CAD build for the part. Positions are in the model's coordinates, mm. Face numbers are marked on the shaded views. Give positions to 0.01 mm unless a question says otherwise; leave off trailing zeros. Loops run counter-clockwise (first coordinate to the right, second up) from the corner with the lowest first, then second, coordinate; pieces in that order, holes last.
Item 1: Saw through at A-A on z = 1.15. Give the cut face in (x, y), plus the area to 3 significant figures.
Item 2: Saw through at B-B on y = -23.5. Give the cut face in (x, z), plus the area to 3 significant figures.
Item 3: Saw through at C-C on x = 16. Give the cut face in (y, z).
Item 4: Mould opens along X. For the marked faces 1 and 2 say: released by +X, released by -X, zero draft, split by the parting line, or undercut.
Item 5: Probe probe 1 along Y at (x, z) = (0, 2.9); probe 2 along Y at (x, z) = (5, 3.5); probe 3 along Y at (x, z) = (0, 4.3). List the from-to ranges inside material, lowest first.
Item 6: Saw through at D-D on y = -32.5. Give the cut face in (x, z), plus the area to 3 significant figures.
Item 7: Drop flat-ended pins along their axis: P1, Ø2, axis at y = -16.5, z = 0.5, coming from the -X side; P2, Ø2, axis at y = -14, z = 1, coming from the +X side; P3, Ø24, axis at x = -12.5, y = -14.5, coming from the +Z side. Give the stop position or say it passes through.
from build123d import *
from build123d import SkipClean  # not in build123d's __all__

# Parameters (mm, degrees)
F0_R      = 39.5
F1_DEPTH  = 2
F2_R      = 37.5
F2_R_2    = 35
F3_DEPTH  = 3
F4_R      = 4.1
F5_DEPTH  = 25
F6_R      = 6
F6_R_2    = 4.1
F7_DEPTH  = 2
F9_DEPTH  = 25
F11_DEPTH = 25


# Not quite as in the source:
# - after a boolean that leaves OpenCascade's solid faulty, fix() repairs it


with BuildPart() as f1:
    # F0 (on Top) → F1 (new body)
    with BuildSketch(Plane.XY):
        Circle(F0_R)
    extrude(amount=F1_DEPTH)

    # F2 (on face) → F3 (join)
    with BuildSketch(Plane.XY.offset(2)):
        Circle(F2_R)
        Circle(F2_R_2, mode=Mode.SUBTRACT)
    extrude(amount=F3_DEPTH)

    # F4 (on face) → F5 (cut)
    with BuildSketch(Plane.XY.offset(2)):
        Circle(F4_R)
    extrude(amount=-F5_DEPTH, mode=Mode.SUBTRACT)

    # F6 (on face) → F7 (join)
    with BuildSketch(Plane.XY.offset(2)):
        Circle(F6_R)
        Circle(F6_R_2, mode=Mode.SUBTRACT)
    extrude(amount=F7_DEPTH)

    # F8 (on face) → F9 (cut)
    with BuildSketch(Plane.XY.offset(2)):
        with BuildLine():
            Line((30.3108891325, 17.5), (0, 35))
            Line((0, 35), (0, 6))
            ThreePointArc((0, 6), (3, 5.1961524227), (5.1961524227, 3))
            Line((5.1961524227, 3), (30.3108891325, 17.5))
        make_face()
        with BuildLine():
            Line((0, -35), (30.3108891325, -17.5))
            Line((30.3108891325, -17.5), (5.1961524227, -3))
            ThreePointArc((5.1961524227, -3), (3, -5.1961524227), (0, -6))
            Line((0, -6), (0, -35))
        make_face()
        with BuildLine():
            ThreePointArc((30.3108891325, 17.5), (17.5, 30.3108891325), (0, 35))
            Line((0, 35), (30.3108891325, 17.5))
        make_face()
        with BuildLine():
            ThreePointArc((0, -35), (17.5, -30.3108891325), (30.3108891325, -17.5))
            Line((30.3108891325, -17.5), (0, -35))
        make_face()
        with BuildLine():
            Line((-5.1961524227, 3), (-30.3108891325, 17.5))
            Line((-30.3108891325, 17.5), (-30.3108891325, -17.5))
            Line((-30.3108891325, -17.5), (-5.1961524227, -3))
            ThreePointArc((-5.1961524227, -3), (-6, 0), (-5.1961524227, 3))
        make_face()
        with BuildLine():
            Line((-30.3108891325, -17.5), (-30.3108891325, 17.5))
            ThreePointArc((-30.3108891325, 17.5), (-35, 0), (-30.3108891325, -17.5))
        make_face()
    with SkipClean():  # cleaning this boolean's faces spoils the solid; the shape is the same uncleaned
        extrude(amount=-F9_DEPTH, mode=Mode.SUBTRACT)

    # F10 (on face) → F11 (cut)
    with BuildSketch(Plane.XY.offset(2)):
        with BuildLine():
            Line((-5, 9.7979589711), (-5, 29.5803989155))
            ThreePointArc((-5, 29.5803989155), (-15, 25.9807621135), (-23.1173769149, 19.1203264767))
            Line((-23.1173769149, 19.1203264767), (-5.9852813742, 9.2291065045))
            ThreePointArc((-5.9852813742, 9.2291065045), (-5.5, 9.5262794416), (-5, 9.7979589711))
        make_face()
        with BuildLine():
            ThreePointArc((10.9852813742, 0.5688524666), (11, 0), (10.9852813742, -0.5688524666))
            Line((10.9852813742, -0.5688524666), (28.1173769149, -10.4600724388))
            ThreePointArc((28.1173769149, -10.4600724388), (30, 0), (28.1173769149, 10.4600724388))
            Line((28.1173769149, 10.4600724388), (10.9852813742, 0.5688524666))
        make_face()
        with BuildLine():
            ThreePointArc((-5, -9.7979589711), (-5.5, -9.5262794416), (-5.9852813742, -9.2291065045))
            Line((-5.9852813742, -9.2291065045), (-23.1173769149, -19.1203264767))
            ThreePointArc((-23.1173769149, -19.1203264767), (-15, -25.9807621135), (-5, -29.5803989155))
            Line((-5, -29.5803989155), (-5, -9.7979589711))
        make_face()
    extrude(amount=-F11_DEPTH, mode=Mode.SUBTRACT)

    add(f1.part.fix(), mode=Mode.REPLACE)


solid = f1.part
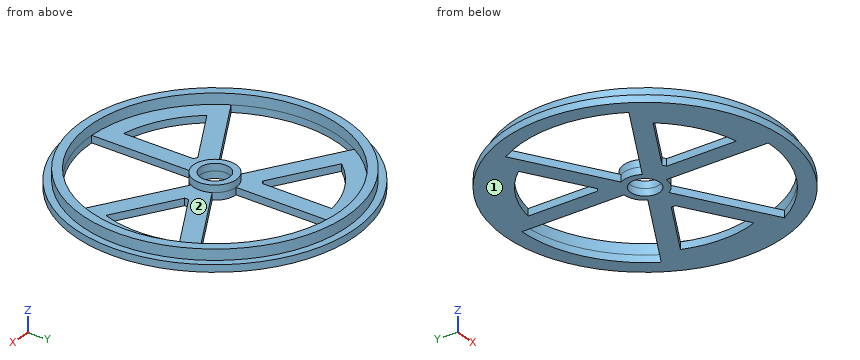
Results below:
1. outline: circle Ø79 at (0, 0); hole (-30.31, -17.5) - (-5.2, -3) arc R6 cw to (-5.2, 3) - (-30.31, 17.5) arc R35 ccw to start; hole (-23.12, -19.12) arc R30 ccw to (-5, -29.58) - (-5, -9.8) arc R11 cw to (-5.99, -9.23) - close; hole (-23.12, 19.12) - (-5.99, 9.23) arc R11 cw to (-5, 9.8) - (-5, 29.58) arc R30 ccw to start; hole circle Ø8.2 at (0, 0); hole (0, -35) arc R35 ccw to (30.31, -17.5) - (5.2, -3) arc R6 cw to (0, -6) - close; hole (0, 6) arc R6 cw to (5.2, 3) - (30.31, 17.5) arc R35 ccw to (0, 35) - close; hole (10.99, -0.57) - (28.12, -10.46) arc R30 ccw to (28.12, 10.46) - (10.99, 0.57) arc R11 cw to start
1. area: 2,340 mm2
2. outline: (-31.75, 0) - (-18.65, 0) - (-18.65, 2) - (-25.94, 2) - (-25.94, 5) - (-29.22, 5) - (-29.22, 2) - (-31.75, 2) - close; (-5, 0) - (0, 0) - (0, 2) - (-5, 2) - close; (25.94, 0) - (31.75, 0) - (31.75, 2) - (29.22, 2) - (29.22, 5) - (25.94, 5) - close
2. area: 67.5 mm2
3. outline: (-36.11, 0) - (-31.13, 0) - (-31.13, 5) - (-33.92, 5) - (-33.92, 2) - (-36.11, 2) - close; (-9.24, 0) - (-3.46, 0) - (-3.46, 2) - (-9.24, 2) - close; (3.46, 0) - (9.24, 0) - (9.24, 2) - (3.46, 2) - close; (31.13, 0) - (36.11, 0) - (36.11, 2) - (33.92, 2) - (33.92, 5) - (31.13, 5) - close
4. face 1: zero draft
4. face 2: undercut
5. probe 1: y = -37.5 to -35, -6 to -4.1, 4.1 to 6, 35 to 37.5
5. probe 2: y = -37.17 to -34.64, -3.32 to 3.32, 34.64 to 37.17
5. probe 3: y = -37.5 to -35, 35 to 37.5
6. outline: (-22.45, 0) - (0, 0) - (0, 2) - (-12.99, 2) - (-12.99, 5) - (-18.71, 5) - (-18.71, 2) - (-22.45, 2) - close; (12.99, 0) - (22.45, 0) - (22.45, 2) - (18.71, 2) - (18.71, 5) - (12.99, 5) - close
6. area: 98.1 mm2
7. P1: stops at x = -36.33
7. P2: stops at x = 37.3
7. P3: stops at z = 2
